Check sheet for the drawn part. Datum: minimum x, y, z corner. Units: mm. A direction names the side the tool comes from. Coordinates: 2 decimals unless noted, no trailing zeros. Order: outer loops, then holes, each group sorted by start corner. A loop starts at its lowest first (then second) coordinate and runs counter-clockwise, first axis right, second up. Notation, with made-up numbers: (59, 8) - (72, 8) arc R26 ccw to (72, 33) - close; hole circle Ø1 at (75.25, 66). An arc over 180 degrees is marked (long way). Answer as CSV lines item,"result". Start each with the question number.
1. Section check B-B (x = 13.5). Record the cut outline in (y, z) (1 decimal).
2. Section check A-A (y = 6). Count the separate pieces of the cut face and the enclosed holes in it.
3. Set-up check for the marked faces 1, 2 and 3: record each of +Z, -Z, +X, -X, +Y, -Y from which the full face is reachable in a straight line by a thin tool's end or side.
4. Material ranges on L1, parallel to X at y = 30, z = 2 (1 decimal); L2, parallel to Z at x = 13, y = 97; L3, parallel to X at y = 83.5, z = 10 (1 decimal), recorded low to high. Write a range as [from, to].
5. Section check C-C (z = 3). Record the cut outline in (x, y) (1 decimal).
6. Go/stop test with flat-tipped pins: pin 1 (11.5 mm diameter, centred on x = 14.5, y = 64.5, fed in from +Z); pin 2 (6 mm diameter, centred on x = 17, y = 87, fed in from -Z); pin 3 (1.8 mm diameter, centred on x = 16.5, z = 11.5, fed in from -Y) (1 decimal); pin 4 (1 mm diameter, centred on x = 1.5, z = 20, fed in from +Y). Record where each tip stops, or that it passes through.
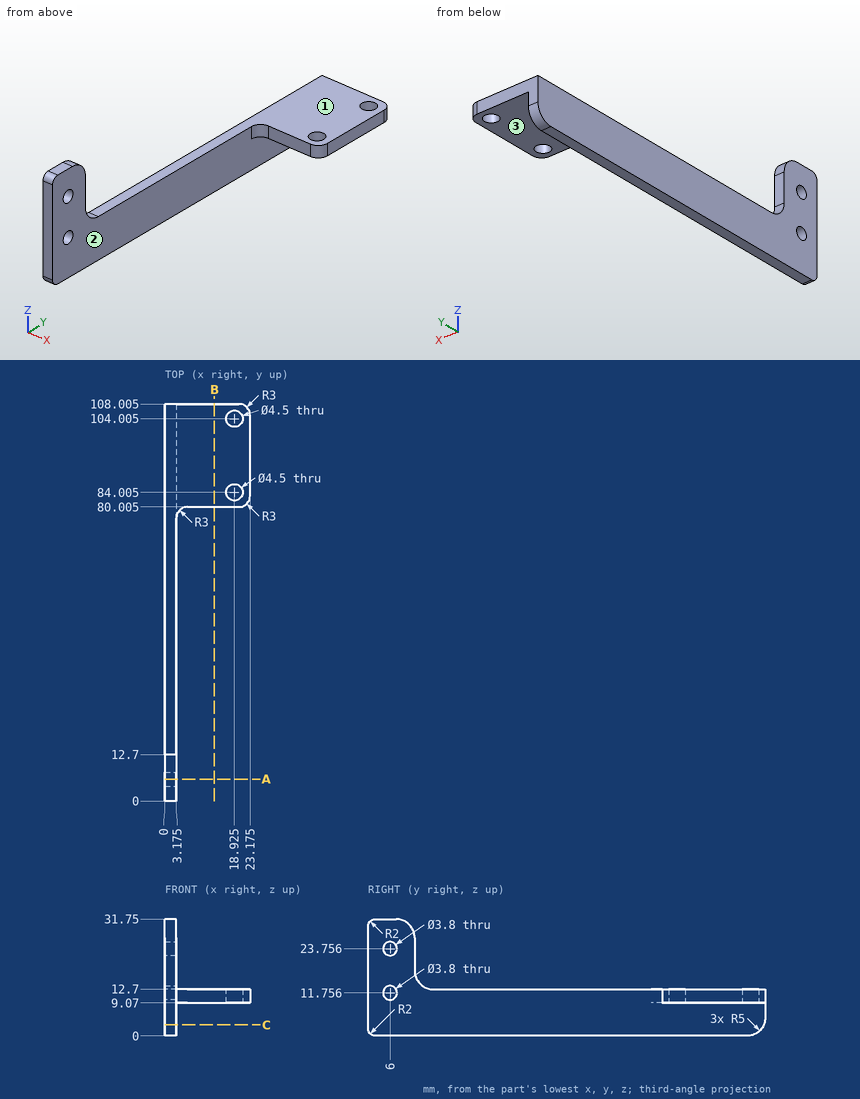
Evaluation:
1,outline,"(80, 9.1) - (108, 9.1) - (108, 12.7) - (80, 12.7) - close"
2,separate pieces,"3"
2,enclosed holes,"0"
3,face 1,"+Z, +X, -X, +Y"
3,face 2,"-Z, +X, -Y"
3,face 3,"-Z, +X, +Y, -Y"
4,L1,"x = [0, 3.2]"
4,L2,"z = [9.07, 12.7]"
4,L3,"x = [0, 16.7], [21.1, 23.2]"
5,outline,"(0, 0) - (3.2, 0) - (3.2, 107.6) - (0, 107.6) - close"
6,pin 1,"passes through"
6,pin 2,"stops at z = 9.07"
6,pin 3,"stops at y = 80"
6,pin 4,"stops at y = 12.7"
